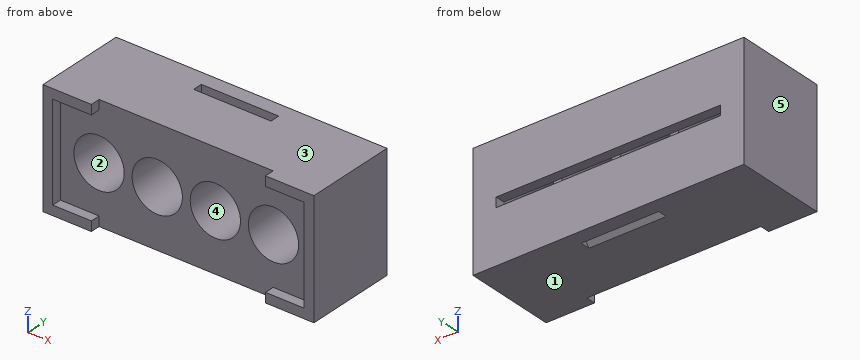
from build123d import *

# Parameters (mm, degrees)
SKICA1_W                 = 28
SKICA1_H                 = 8.5
P_IDAT_VYSUNUT_M1_DEPTH  = 12
SKICA3_R                 = 2.6
ODEBRAT_VYSUNUT_M2_DEPTH = 7.5
SKICA4_W                 = 23.2
SKICA4_H                 = 1
ODEBRAT_VYSUNUT_M3_DEPTH = 1
SKICA5_W                 = 5
SKICA5_H                 = 12
P_IDAT_VYSUNUT_M2_DEPTH  = 1
SKICA6_W                 = 4
SKICA6_H                 = 10
ODEBRAT_VYSUNUT_M4_DEPTH = 1
ODEBRAT_START            = -10
ODEBRAT_VYSUNUT_M5_DEPTH = 8


with BuildPart() as part:
    # Skica1 → Přidat vysunutím1 (new body)
    with BuildSketch(Plane.XY):
        with Locations((-32.656744291, -2.464704976)):
            Rectangle(SKICA1_W, SKICA1_H)
    extrude(amount=P_IDAT_VYSUNUT_M1_DEPTH)

    # Skica3 → Odebrat vysunutím2 (cut)
    with BuildSketch(Plane(origin=(0, -6.714704976, 0), x_dir=(-1, 0, 0), z_dir=(0, -1, 0))):
        with Locations((41.656744291, -6)):
            Circle(SKICA3_R)
        with Locations((35.646744291, -6)):
            Circle(SKICA3_R)
        with Locations((29.636744291, -6)):
            Circle(SKICA3_R)
        with Locations((23.626744291, -6)):
            Circle(SKICA3_R)
    extrude(amount=-ODEBRAT_VYSUNUT_M2_DEPTH, mode=Mode.SUBTRACT)

    # Skica4 → Odebrat vysunutím3 (cut)
    with BuildSketch(Plane(origin=(0, 1.785295024, 0), x_dir=(1, 0, 0), z_dir=(0, 1, 0))):
        with Locations((-32.656744291, -6)):
            Rectangle(SKICA4_W, SKICA4_H)
    extrude(amount=-ODEBRAT_VYSUNUT_M3_DEPTH, mode=Mode.SUBTRACT)

    # Skica5 → Přidat vysunutím2 (add)
    with BuildSketch(Plane(origin=(0, -6.714704976, 0), x_dir=(-1, 0, 0), z_dir=(0, -1, 0))):
        with Locations((44.156744291, -6)):
            Rectangle(SKICA5_W, SKICA5_H)
        with Locations((21.156744291, -6)):
            Rectangle(SKICA5_W, SKICA5_H)
    extrude(amount=P_IDAT_VYSUNUT_M2_DEPTH)

    # Skica6 → Odebrat vysunutím4 (cut)
    with BuildSketch(Plane(origin=(0, -7.714704976, 0), x_dir=(-1, 0, 0), z_dir=(0, -1, 0))):
        with Locations((43.656744291, -6)):
            Rectangle(SKICA6_W, SKICA6_H)
        with Locations((21.656744291, -6)):
            Rectangle(SKICA6_W, SKICA6_H)
    extrude(amount=-ODEBRAT_VYSUNUT_M4_DEPTH, mode=Mode.SUBTRACT)

    # Skica9 → Odebrat vysunutím5 (cut)
    with BuildSketch(Plane(origin=(-18.656744291, 0, 0), x_dir=(0, 0, -1), z_dir=(1, 0, 0)).offset(ODEBRAT_START)):
        Polygon((-12, 0.285295024), (-11, 0.285295024), (-12, -0.714704976), align=None)
        Polygon((0, 0.285295024), (-1, 0.285295024), (0, -0.714704976), align=None)
    extrude(amount=-ODEBRAT_VYSUNUT_M5_DEPTH, mode=Mode.SUBTRACT)


solid = part.part
The listing builds one solid part. Answer for the finished solid, in the listing's coordinates (mm). Face numbers are marked on the shaded views. A direction names the side the tool comes from. Coordinates: 2 decimals unless noted, no trailing zeros. Order: outer loops, then holes, each group sorted by start corner. A loop starts at its lowest first (then second) coordinate and runs counter-clockwise, first axis right, second up.
Q1. Which of the six approach directions +Z, -Z, +X, -X, +Y, -Y give full straight-line access (tool end or side, diameter ignored) to the marked faces 4 and 5?
Q2. A cutting plane is placed at D-D, the plane z = 9.25. Write down the section's boundary in (x, y).
Q3. A cutting plane is placed at B-B, the plane x = -21.75. Write down the section's boundary in (y, z).
Q4. Given P1, Ø1.1, axis at x = -36, z = 7.5, coming from the -Y side; P2, Ø1.1, axis at x = -24.5, z = 4, coming from the -Y side; P3, Ø5, axis at x = -22.5, z = 10, coming from the -Y side; P4, Ø0.7, axis at x = -39, z = 6, coming from the +Y side, each flat-ended and moving along its own axis, determine where each tip first touches the part or whether it passes through.
Q5. A cutting plane is placed at C-C, the plane y = -3.5. Write down the section's boundary in (x, z).
Q6. Consider line 1 (X direction, y = -4.75, z = 6.5); line 2 (X direction, y = -2.75, z = 6); line 3 (X direction, y = -6.75, z = 2). Determine where each line is inside the solid, lowest interval first.
Q7. For a pull along Z with two mould halves and no side action, classify the marked faces 1, 2 and 3 as pulls with the +Z half, pulls with the -Z half, needs draft (parallel to the pull), parting line crosses it, or undercut.
Q8. A cutting plane is placed at A-A, the plane y = -7. Write down the section's boundary in (x, z), and give its area (3 significant figures).
Answers follow:
1. face 4: -Y
1. face 5: +Z, -Z, -X, +Y, -Y
2. outline: (-46.66, -7.71) - (-45.66, -7.71) - (-45.66, -6.71) - (-19.66, -6.71) - (-19.66, -7.71) - (-18.66, -7.71) - (-18.66, 1.79) - (-46.66, 1.79) - close
3. outline: (-7.71, 0) - (1.79, 0) - (1.79, 5.5) - (0.79, 5.5) - (0.79, 4.2) - (-6.71, 4.2) - (-6.71, 1) - (-7.71, 1) - close; (-7.71, 11) - (-6.71, 11) - (-6.71, 7.8) - (0.79, 7.8) - (0.79, 6.5) - (1.79, 6.5) - (1.79, 12) - (-7.71, 12) - close
4. P1: stops at y = 0.79
4. P2: stops at y = -6.71
4. P3: stops at y = -7.71
4. P4: stops at y = 0.79
5. outline: (-46.66, 0) - (-18.66, 0) - (-18.66, 12) - (-46.66, 12) - close; hole circle Ø5.2 at (-41.66, 6); hole circle Ø5.2 at (-35.65, 6); hole circle Ø5.2 at (-29.64, 6); hole circle Ø5.2 at (-23.63, 6)
6. line 1: x = -46.66 to -44.21, -39.11 to -38.2, -33.1 to -32.19, -27.09 to -26.18, -21.08 to -18.66
6. line 2: x = -46.66 to -44.26, -39.06 to -38.25, -33.05 to -32.24, -27.04 to -26.23, -21.03 to -18.66
6. line 3: x = -46.66 to -45.66, -19.66 to -18.66
7. face 1: pulls with the -Z half
7. face 2: undercut
7. face 3: pulls with the +Z half
8. outline: (-46.66, 0) - (-41.66, 0) - (-41.66, 1) - (-45.66, 1) - (-45.66, 11) - (-41.66, 11) - (-41.66, 12) - (-46.66, 12) - close; (-23.66, 0) - (-18.66, 0) - (-18.66, 12) - (-23.66, 12) - (-23.66, 11) - (-19.66, 11) - (-19.66, 1) - (-23.66, 1) - close
8. area: 40.0 mm2
